Here's how the part is built. I have some questions about the finished solid (model axes, mm). Face numbers are marked on the shaded views. A direction names the side the tool comes from. Round coordinates to 2 decimals unless told otherwise and drop trailing zeros. Loops run counter-clockwise (first coordinate to the right, second up) from the corner with the lowest first, then second, coordinate; pieces in that order, holes last. Notation, with made-up numbers: M 47,46.25 L 53,46.25 A6 cw 53,56.25 Z; hole C 73,19 d6. An arc over 180 degrees is marked long. Answer as CSV lines item,"result".
```python
from build123d import *

# Parameters (mm, degrees)
SALIENTE_EXTRUIR1_DEPTH                              = 15
CROQUIS2_R                                           = 6
CORTAR_EXTRUIR1_DEPTH                                = 16
PERFORADOR_PARA_ROSCAR_PARA_MACHO_DE_ROS_D           = 3.3
PERFORADOR_PARA_ROSCAR_PARA_MACHO_DE_ROS_DEPTH       = 7
PERFORADOR_PARA_ROSCAR_PARA_MACHO_DE_ROS_TIP         = 0.991420021
CROQUIS9_W                                           = 80
CROQUIS9_H                                           = 38
CORTAR_EXTRUIR2_DEPTH                                = 2
TALADROS_DE_ESPIGA_DE_4_0MM1_D                       = 4
TALADROS_DE_ESPIGA_DE_4_0MM1_DEPTH                   = 17
TALADROS_DE_ESPIGA_DE_4_0MM1_TIP                     = 1.201721238
TALADRO_ROSCADO_M41_D                                = 3.3
TALADRO_ROSCADO_M41_DEPTH                            = 11.5
TALADRO_ROSCADO_M41_TIP                              = 0.991420021
REFRENTADO_PARA_TORNILLO_CON_CABEZA_HUEC_D           = 4.5
REFRENTADO_PARA_TORNILLO_CON_CABEZA_HUEC_CBORE_D     = 8
REFRENTADO_PARA_TORNILLO_CON_CABEZA_HUEC_CBORE_DEPTH = 4.4
TALADROS_DE_ESPIGA_DE_4_0MM2_D                       = 4


with BuildPart() as part:
    # Croquis1 → Saliente-Extruir1 (new body)
    with BuildSketch(Plane.XY):
        with BuildLine():
            Line((80, 0), (80, 40))
            Line((80, 40), (9.228509485, 290.860669242))
            ThreePointArc((9.228509485, 290.860669242), (-5.12786552, 311.893782856), (-29.268839302, 320))
            Line((-29.268839302, 320), (-50, 320))
            Line((-50, 320), (-50, 220))
            Line((-50, 220), (-0.751325607, 45.430334621))
            ThreePointArc((-0.751325607, 45.430334621), (-0.1887218, 42.741031935), (0, 40))
            Line((0, 40), (0, 0))
            Line((0, 0), (80, 0))
        make_face()
    extrude(amount=SALIENTE_EXTRUIR1_DEPTH)

    # Croquis2 → Cortar-Extruir1 (cut, through all)
    with BuildSketch(Plane(origin=(0, 0, 0), x_dir=(-1, 0, 0), z_dir=(0, 0, -1))):
        with Locations((39, 280)):
            Circle(CROQUIS2_R)
    extrude(amount=-CORTAR_EXTRUIR1_DEPTH, mode=Mode.SUBTRACT)

    # Perforador para roscar para macho de roscar para M44
    with Locations(Plane(origin=(0, 0, 0), x_dir=(-1, 0, 0), z_dir=(0, 0, -1))):
        with Locations((39, 261.75), (39, 298.25)):
            Hole(PERFORADOR_PARA_ROSCAR_PARA_MACHO_DE_ROS_D / 2, depth=PERFORADOR_PARA_ROSCAR_PARA_MACHO_DE_ROS_DEPTH)
            with Locations((0, 0, -(PERFORADOR_PARA_ROSCAR_PARA_MACHO_DE_ROS_DEPTH + PERFORADOR_PARA_ROSCAR_PARA_MACHO_DE_ROS_TIP / 2))):  # 118° drill point
                Cone(0, PERFORADOR_PARA_ROSCAR_PARA_MACHO_DE_ROS_D / 2, PERFORADOR_PARA_ROSCAR_PARA_MACHO_DE_ROS_TIP, mode=Mode.SUBTRACT)

    # Croquis9 → Cortar-Extruir2 (cut)
    with BuildSketch(Plane.XY.offset(15)):
        with Locations((40, 19)):
            Rectangle(CROQUIS9_W, CROQUIS9_H)
    extrude(amount=-CORTAR_EXTRUIR2_DEPTH, mode=Mode.SUBTRACT)

    # Taladros de espiga de Ø4.0mm1
    with Locations(Plane.ZY.offset(50)):
        with Locations((6, 304), (6, 256)):
            Hole(TALADROS_DE_ESPIGA_DE_4_0MM1_D / 2, depth=TALADROS_DE_ESPIGA_DE_4_0MM1_DEPTH)
            with Locations((0, 0, -(TALADROS_DE_ESPIGA_DE_4_0MM1_DEPTH + TALADROS_DE_ESPIGA_DE_4_0MM1_TIP / 2))):  # 118° drill point
                Cone(0, TALADROS_DE_ESPIGA_DE_4_0MM1_D / 2, TALADROS_DE_ESPIGA_DE_4_0MM1_TIP, mode=Mode.SUBTRACT)

    # Taladro roscado M41
    with Locations(Plane.ZY.offset(50)):
        with Locations((6, 312), (6, 248), (6, 291), (6, 269)):
            Hole(TALADRO_ROSCADO_M41_D / 2, depth=TALADRO_ROSCADO_M41_DEPTH)
            with Locations((0, 0, -(TALADRO_ROSCADO_M41_DEPTH + TALADRO_ROSCADO_M41_TIP / 2))):  # 118° drill point
                Cone(0, TALADRO_ROSCADO_M41_D / 2, TALADRO_ROSCADO_M41_TIP, mode=Mode.SUBTRACT)

    # Refrentado para tornillo con cabeza hueca de M41 (through all)
    with Locations(Plane(origin=(0, 0, 0), x_dir=(-1, 0, 0), z_dir=(0, 0, -1))):
        with Locations((-57, 7), (-57, 33), (-31, 33), (-31, 7)):
            CounterBoreHole(REFRENTADO_PARA_TORNILLO_CON_CABEZA_HUEC_D / 2, REFRENTADO_PARA_TORNILLO_CON_CABEZA_HUEC_CBORE_D / 2, REFRENTADO_PARA_TORNILLO_CON_CABEZA_HUEC_CBORE_DEPTH)

    # Taladros de espiga de Ø4.0mm2 (through all)
    with Locations(Plane(origin=(0, 0, 0), x_dir=(-1, 0, 0), z_dir=(0, 0, -1))):
        with Locations((-44, 32), (-44, 6)):
            Hole(TALADROS_DE_ESPIGA_DE_4_0MM2_D / 2)


solid = part.part
```
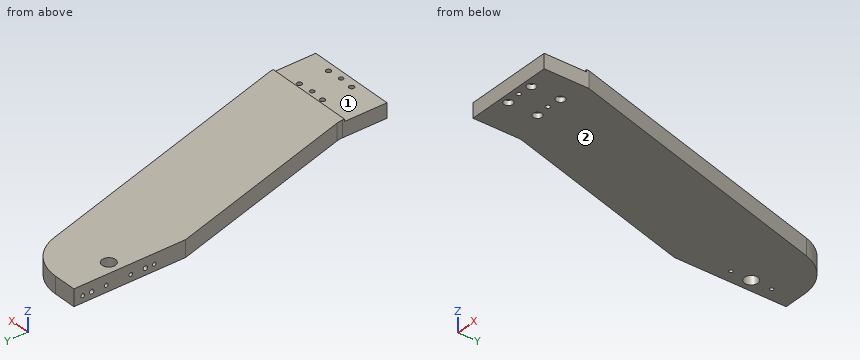
1. For P1, Ø1, axis at y = 195, z = 5.5, coming from the +X side; P2, Ø1, axis at x = 28.5, z = 14, coming from the -Y side; P3, Ø4, axis at x = 57, y = 33, coming from the +Z side; P4, Ø6.5, axis at x = 57, y = 7, coming from the -Z side, each with a flat end and sliding along its axis, tell me the tip position at first contact or that it passes through.
Evaluation:
P1,"stops at x = 36.41"
P2,"stops at y = 38"
P3,"passes through"
P4,"stops at z = 4.4"
2. I want a section at B-B, the plane x = -15. Please give me the cut outline in (y, z).
Evaluation:
outline,"M 95.94,0 L 317.37,0 L 317.37,15 L 95.94,15 Z"
3. Which directions (+Z, -Z, +X, -X, +Y, -Y) give clear straight access to the entire face, cutting with the end or side of a thin tool? Please do the marked faces 1 and 2.
Evaluation:
face 1,"+Z, +X, -X, -Y"
face 2,"-Z, +X, -X, +Y, -Y"
4. I want a section at A-A, the plane y = 73.5. Please give me the cut outline in (x, z), and give its area (3 significant figures).
Evaluation:
outline,"M -8.67,0 L 70.55,0 L 70.55,15 L -8.67,15 Z"
area,"1,190 mm²"
5. If I drill on line 1 (Z direction, x = -37, y = 304); line 2 (Z direction, x = 54, y = 25.5); line 3 (X direction, y = 297.5, z = 10.5), over which ranges is the centre line in solid material (lowest first)? Write a range as [from, to].
Evaluation:
line 1,"z = [0, 4], [8, 15]"
line 2,"z = [0, 13]"
line 3,"x = [-50, 6.7]"
